For this review, use the dimensioned drawing (mm, ordinates from the lowest corner) and the shaded views. A direction names the side the tool comes from. Give positions to 0.01 mm unless a question says otherwise; leave off trailing zeros. Loops run counter-clockwise (first coordinate to the right, second up) from the corner with the lowest first, then second, coordinate; pieces in that order, holes last. Notation, with made-up numbers: M 43,38.25 L 91,38.25 A13 ccw 91,47.25 Z; hole C 48,28.5 d4. An arc over 180 degrees is marked long. Use CSV: the item, a comma, the result in double quotes.
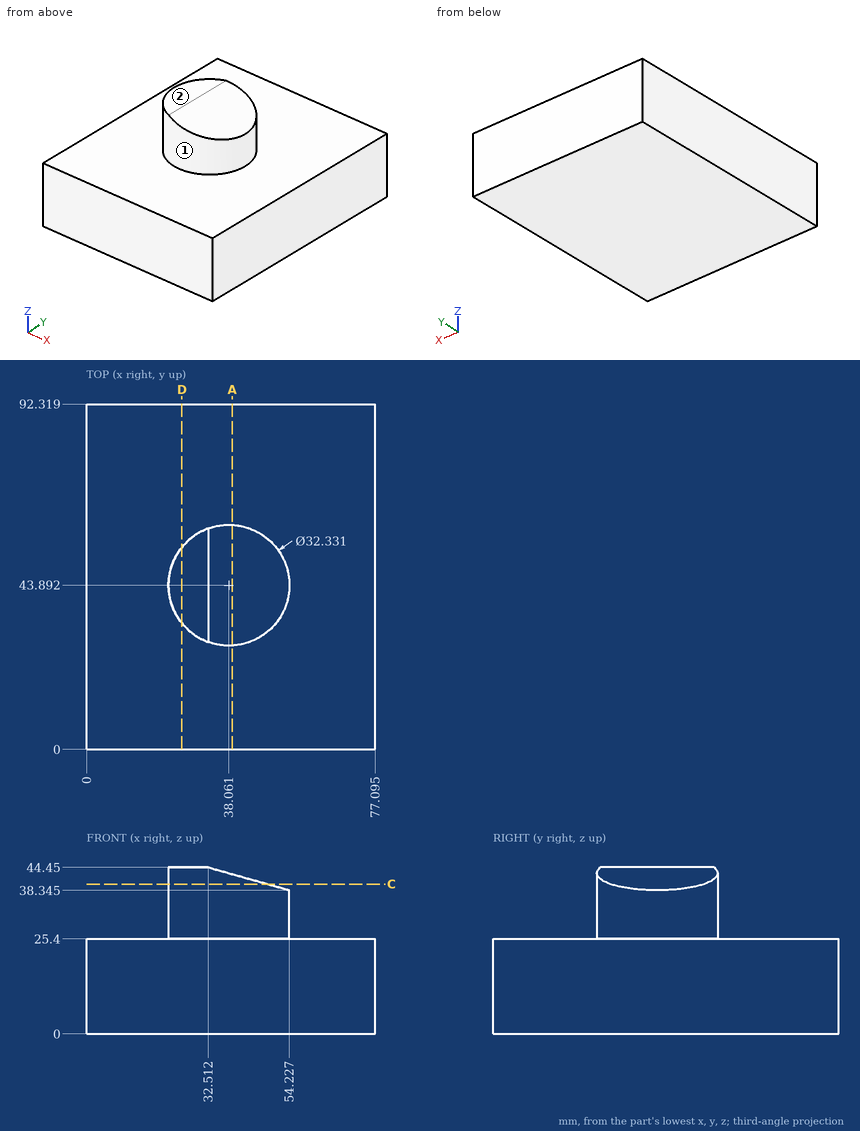
(1) Machinability: for the marked faces 1 and 2, which of the approach directions +Z, -Z, +X, -X, +Y, -Y give a long, thin tool a straight path to every point of the face, cutting with its end or side? Answer none if there is none.
A:
face 1,"+Z"
face 2,"+Z, +X, -X, +Y, -Y"
(2) Clearance check with flat-ended pins moving along their axes: P1, Ø4, axis at x = 46, y = 55.5, coming from the +Z side; P2, Ø12, axis at x = 67.5, y = 20, coming from the -Z side; P3, Ø10, axis at x = 28, y = 12.5, coming from the +Z side. State where each tip first meets the part, or that it passes through.
A:
P1,"z = 41.22"
P2,"z = 0"
P3,"z = 25.4"
(3) We need section A-A on x = 39. State the section outline as (y, z) points, then the cut area to 3 significant figures.
A:
outline,"M 0,0 L 92.32,0 L 92.32,25.4 L 60.03,25.4 L 60.03,42.63 L 27.75,42.63 L 27.75,25.4 L 0,25.4 Z"
area,"2,900 mm²"
(4) We need section D-D on x = 25.5. State the section outline as (y, z) points.
A:
outline,"M 0,0 L 92.32,0 L 92.32,25.4 L 54.07,25.4 L 54.07,44.45 L 33.72,44.45 L 33.72,25.4 L 0,25.4 Z"
(5) We need section C-C on z = 40. State the section outline as (x, y) points (1 decimal).
A:
outline,"M 48.3,31.4 L 48.3,56.4 A16.2 ccw long Z"
(6) Wall thickness on line 1 along Z through (x, y) = (65, 23); line 2 along X through (y, z) = (50, 30) (1 decimal); line 3 along Y through (x, z) = (27.5, 43) (1 decimal): over which ranges is each line inside the solid? List them lowest first. Write a range as [from, to].
A:
line 1,"[0, 25.4]"
line 2,"[23.1, 53]"
line 3,"[31.7, 56.1]"
